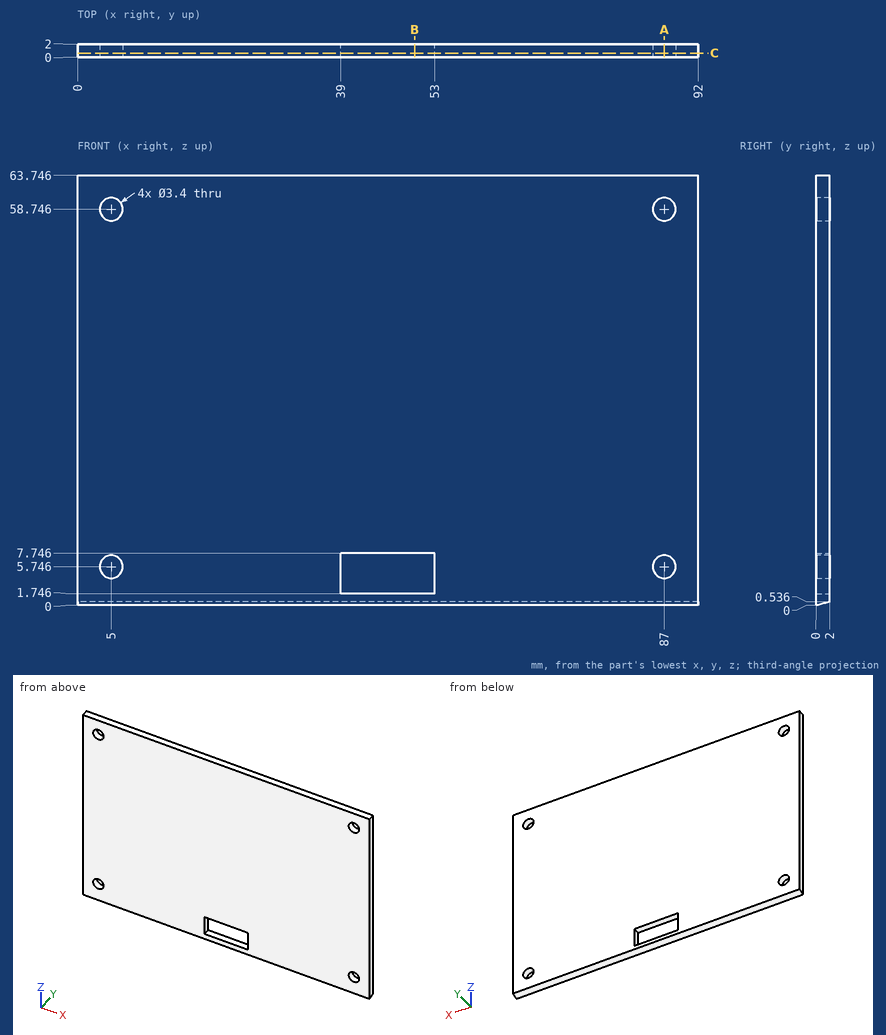
Study the drawing (mm; zero at the part's minimum x, y, z) and answer. Round coordinates to 2 decimals unless told otherwise and drop trailing zeros. Write each loop counter-clockwise with the first axis right and the second up, starting at its lowest first coordinate (ties: lowest second). Pieces come first, ordered by that corner, then holes.
Q1. Find section A-A on x = 87. Determine the outline of the cut face in (y, z).
Values:
outline: (0, 0) - (2, 0.54) - (2, 4.05) - (0, 4.05) - close; (0, 7.45) - (2, 7.45) - (2, 57.05) - (0, 57.05) - close; (0, 60.45) - (2, 60.45) - (2, 63.75) - (0, 63.75) - close
Q2. Straight lines are drawn through the part: line 1 (Z direction, x = 87, y = 0.6); line 2 (Z direction, x = 41.5, y = 0.3); line 3 (Z direction, x = 81, y = 1). For each, find the intervals that lie inside material, in ascending order.
Values:
line 1: z = 0.16 to 4.05, 7.45 to 57.05, 60.45 to 63.75
line 2: z = 0.08 to 1.75, 7.75 to 63.75
line 3: z = 0.27 to 63.75
Q3. Find section C-C on y = 0.65. Determine the outline of the cut face in (x, z), and give its area (3 significant figures).
Values:
outline: (0, 0.17) - (92, 0.17) - (92, 63.75) - (0, 63.75) - close; hole circle Ø3.4 at (5, 5.75); hole circle Ø3.4 at (5, 58.75); hole (39, 1.75) - (53, 1.75) - (53, 7.75) - (39, 7.75) - close; hole circle Ø3.4 at (87, 5.75); hole circle Ø3.4 at (87, 58.75)
area: 5,730 mm2
Q4. Find section B-B on x = 50. Determine the outline of the cut face in (y, z).
Values:
outline: (0, 0) - (2, 0.54) - (2, 1.75) - (0, 1.75) - close; (0, 7.75) - (2, 7.75) - (2, 63.75) - (0, 63.75) - close
Q5. Flat-ended cylindrical pins translate along their axes: P1, Ø0.6, axis at x = 45, y = 1.5, coming from the -Z side; P2, Ø2.5, axis at x = 5, z = 5.75, coming from the +Y side; P3, Ø1, axis at x = 17, y = 1, coming from the -Z side. Find the tip coordinate at first contact, or state that the pin passes through.
Values:
P1: stops at z = 0.32
P2: passes through
P3: stops at z = 0.13
